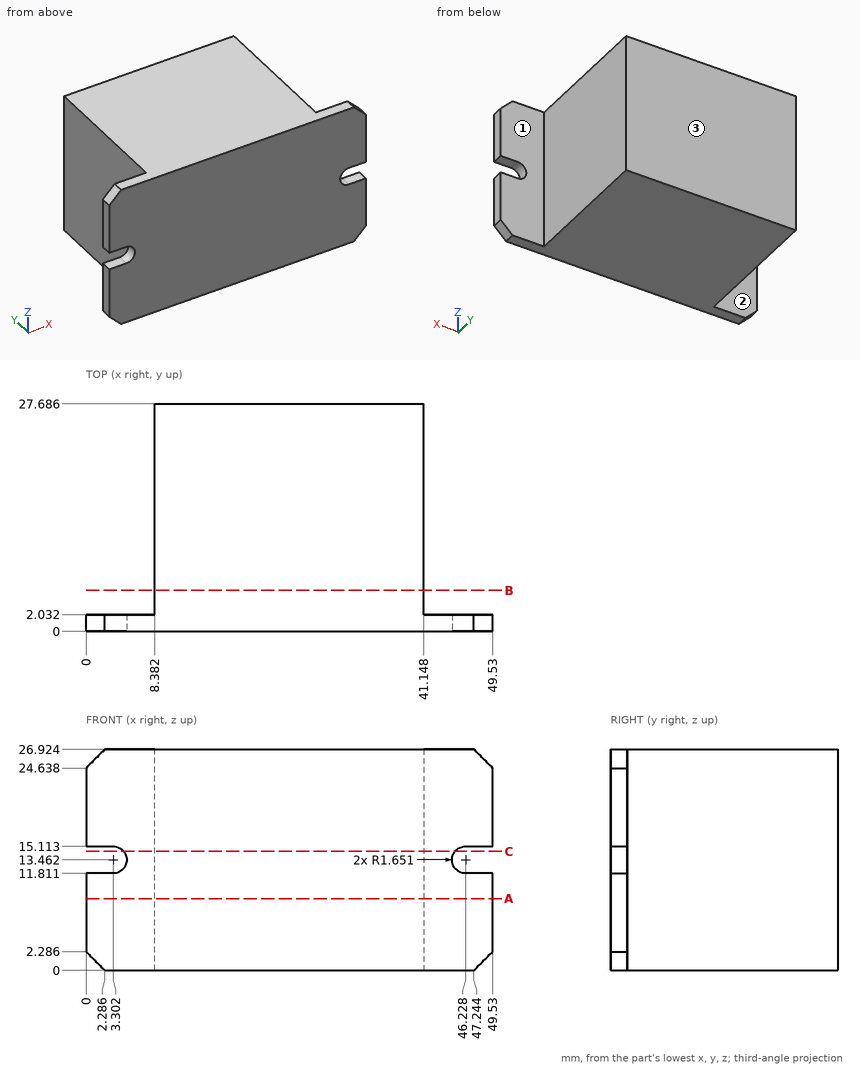
Source: three-view drawing plus pictorial views. Frame: mm from the lowest corner of the part. A direction names the side the tool comes from. Give positions to 0.01 mm unless a question says otherwise; leave off trailing zeros. Write each loop counter-clockwise with the first axis right and the second up, starting at its lowest first coordinate (ties: lowest second). Pieces come first, ordered by that corner, then holes.
(1) Cut plane C-C, the plane z = 14.5. Return loops of the section in (x, y).
(2) Cut plane B-B, the plane y = 5. Return loops of the section in (x, z), then the cut area to 3 significant figures.
(3) First-contact query: P1, Ø4, axis at y = 18, z = 18, coming from the +X side; P2, Ø2.5, axis at x = 44, z = 11, coming from the +Y side; P3, Ø0.6, axis at x = 48, y = 1.5, coming from the -Z side. Flat tips, straight axial feed; report the tip coordinate or a pass-through.
(4) Cut plane A-A, the plane z = 8.75. Return loops of the section in (x, y).
(5) Ray query, line 1 (X direction, y = 2.25, z = 10.75); line 2 (Y direction, x = 5, z = 10.25). Return the intervals inside material, ascending.
(6) Access query for the marked faces 1, 2 and 3. Directions: +Z, -Z, +X, -X, +Y, -Y. A direction counts if a zero-diameter tool reaches every point of the face in a straight line with its end or side. Return the directions, or none.
Values follow:
1. outline: (4.59, 0) - (44.94, 0) - (44.94, 2.03) - (41.15, 2.03) - (41.15, 27.69) - (8.38, 27.69) - (8.38, 2.03) - (4.59, 2.03) - close
2. outline: (8.38, 0) - (41.15, 0) - (41.15, 26.92) - (8.38, 26.92) - close
2. area: 882 mm2
3. P1: stops at x = 41.15
3. P2: stops at y = 2.03
3. P3: stops at z = 0.46
4. outline: (0, 0) - (49.53, 0) - (49.53, 2.03) - (41.15, 2.03) - (41.15, 27.69) - (8.38, 27.69) - (8.38, 2.03) - (0, 2.03) - close
5. line 1: x = 8.38 to 41.15
5. line 2: y = 0 to 2.03
6. face 1: +Z, -Z, +X, +Y
6. face 2: +Z, -Z, -X, +Y
6. face 3: +Z, -Z, +X, -X, +Y
